Autodesk Inventor part; units mm, degrees
ref_plane "YZ Plane" through (0, 0, 0) normal (1, 0, 0) x (0, 1, 0)
ref_plane "XZ Plane" through (0, 0, 0) normal (0, 1, 0) x (-1, 0, 0)
ref_plane "XY Plane" through (0, 0, 0) normal (0, 0, 1) x (1, 0, 0)
ref_plane "Plano de trabajo1" through (0, 3, 0) normal (0, 1, 0) x (1, 0, 0)
ref_plane "Plano de trabajo2" through (4.2498, 73, -5.25) normal (0, 1, 0) x (1, 0, 0)
sketch "Boceto3" plane through (4.2498, 73, -5.25) normal (0, 1, 0) x (1, 0, 0)
  line L0 (37.7502, 51.75) -> (40.7502, 51.75)
  line L1 (-7.2498, -8.25) -> (40.7502, -8.25)
  line L2 (40.7502, -8.25) -> (40.7502, 51.75)
  line L3 (40.7502, 51.75) -> (-7.2498, 51.75)
  line L4 (-7.2498, 51.75) -> (-7.2498, -8.25)
  circle A0 centre (33.5, 43.5) radius 1.25
  circle A1 centre (33.5, 0) radius 1.25
  circle A2 centre (0, 43.5) radius 1.25
  circle A3 centre (0, 0) radius 1.25
  point P0 (-4.2498, -5.25)
  point P1 (37.7502, -5.25)
  point P2 (37.7502, 48.75)
  dimension "d39" = 2.5
  dimension "d40" = 2.5
  dimension "d41" = 2.5
  dimension "d42" = 2.5
ref_plane "Plano de trabajo3" through (4.2498, 73, -5.25) normal (0, -1, 0) x (1, 0, 0)
sketch "Boceto5" plane through (4.2498, 73, -5.25) normal (0, -1, 0) x (1, 0, 0)
  line L0 (-4.2498, 5.25) -> (-4.2498, -48.75)
  line L1 (-4.2498, 5.25) -> (-4.2498, -48.75)
  line L2 (37.7502, -48.75) -> (37.7502, 5.25)
  line L3 (37.7502, 5.25) -> (37.7502, 8.25)
  line L4 (37.7502, -48.75) -> (37.7502, -51.75)
  line L5 (-4.2498, 5.25) -> (-7.2498, 5.25)
  line L6 (-4.2498, -48.75) -> (-7.2498, -48.75)
  line L7 (37.7502, -48.75) -> (40.7502, -48.75)
  line L8 (37.7502, 5.25) -> (40.7502, 5.25)
  line L9 (40.7502, 5.25) -> (40.7502, -48.75)
  line L10 (40.7502, -51.75) -> (40.7502, 8.25)
  line L11 (-7.2498, -48.75) -> (-7.2498, 5.25)
  line L12 (-7.2498, 8.25) -> (-7.2498, -51.75)
extrude "Extrusión5" add sketch "Boceto5" along normal blind 67.5
extrude "Extrusión6" add sketch "Boceto3" along normal blind 3
sketch "Boceto6" plane through (4.2498, 76, -5.25) normal (0, 1, 0) x (1, 0, 0)
  circle A0 centre (0, 43.5) radius 1.25
  circle A1 centre (0, 43.5) radius 1.25
  circle A2 centre (33.5, 43.5) radius 1.25
  circle A3 centre (33.5, 43.5) radius 1.25
  circle A4 centre (33.5, 0) radius 1.25
  circle A5 centre (33.5, 0) radius 1.25
  circle A6 centre (0, 0) radius 1.25
  point P0 (-4.2498, -5.25)
extrude "Extrusión7" add sketch "Boceto6" against normal blind 3
sketch "Boceto8" plane through (45, 5.5, 0) normal (1, 0, 0) x (0, 0, -1)
  line L0 (0, 0) -> (54, 0)
  line L1 (0, 0) -> (54, 0)
  line L2 (54, 0) -> (54, 1.5)
  line L3 (54, 1.5) -> (0, 1.5)
  line L4 (0, 67.5) -> (0, 0)
  line L5 (0, 0) -> (0, 1.5)
  line L6 (54, 1.5) -> (54, 21.5)
  line L7 (54, 21.5) -> (54, 22.5)
  line L8 (54, 22.5) -> (0, 22.5)
  line L9 (0, 22.5) -> (0, 24)
  line L10 (0, 24) -> (54, 24)
  line L11 (54, 22.5) -> (54, 24)
  line L12 (54, 24) -> (54, 45)
  line L13 (54, 67.5) -> (54, 0)
  line L14 (54, 45) -> (0, 45)
  line L15 (0, 45) -> (0, 46.5)
  line L16 (0, 46.5) -> (54, 46.5)
  line L17 (54, 45) -> (54, 46.5)
  line L18 (54, 67.5) -> (0, 67.5)
  line L19 (54, 46.5) -> (54, 67.5)
  point P0 (0, -5.5)
  dimension "d54" = 1.5
  dimension "d55" = 20
  dimension "d60" = 1
  dimension "d61" = 1.5
  dimension "d62" = 21
  dimension "d63" = 1.5
extrude "Extrusión8" add sketch "Boceto8" against normal blind 47.25 contours L4 L3 L2 L0 | L4 L10 L11 L8 | L4 L16 L13 L14
sketch "Boceto9" plane through (-3, 5.5, 0) normal (0, 0, 1) x (1, 0, 0)
  line L0 (3, 67.5) -> (3, 46.5)
  line L1 (3, 46.5) -> (3, 52.5)
  line L2 (3, 52.5) -> (45, 52.5)
  line L3 (45, 67.5) -> (45, 46.5)
  line L4 (45, 52.5) -> (45, 46.5)
  line L5 (45, 46.5) -> (3, 46.5)
  line L6 (45, 46.5) -> (3, 46.5)
  line L7 (45, 45) -> (45, 24)
  line L8 (3, 24) -> (45, 24)
  line L9 (45, 24) -> (45, 30)
  line L10 (45, 30) -> (3, 30)
  line L11 (3, 30) -> (3, 24)
  line L12 (45, 22.5) -> (45, 1.5)
  line L13 (3, 2) -> (3, 1.5)
  line L14 (45, 1.5) -> (3, 1.5)
  line L15 (3, 1.5) -> (45, 1.5)
  line L16 (45, 1.5) -> (45, 7.5)
  line L17 (45, 22.5) -> (45, 1.5)
  line L18 (45, 7.5) -> (3, 7.5)
  line L19 (45, 7.5) -> (45, 1.5)
  line L20 (3, 1.5) -> (3, 7.5)
  line L21 (3, 22.5) -> (3, 1.5)
  point P0 (3, -5.5)
  point P1 (45, 8)
  point P2 (45, 2)
  dimension "d66" = 6
  dimension "d70" = 6
extrude "Extrusión10" add sketch "Boceto9" along normal blind 1.5
sketch "Boceto11" plane through (-3, 5.5, 0) normal (0, 0, 1) x (1, 0, 0)
  line L0 (48, 0) -> (0, 0)
  line L1 (48, 0) -> (0, 0)
  line L2 (0, 0) -> (0, 67.5)
  line L3 (3, 67.5) -> (3, 52.5)
  line L4 (0, 67.5) -> (3, 67.5)
  line L5 (3, 67.5) -> (3, 46.5)
  line L6 (45, 46.5) -> (3, 46.5)
  line L7 (3, 46.5) -> (45, 46.5)
  line L8 (45, 67.5) -> (45, 52.5)
  line L9 (45, 46.5) -> (45, 67.5)
  line L10 (48, 67.5) -> (45, 67.5)
  line L11 (45, 67.5) -> (48, 67.5)
  line L12 (48, 67.5) -> (48, 0)
  line L13 (3, 7.5) -> (3, 1.5)
  line L14 (3, 22.5) -> (3, 7.5)
  line L15 (3, 7.5) -> (3, 22.5)
  line L16 (3, 22.5) -> (45, 22.5)
  line L17 (45, 22.5) -> (45, 1.5)
  line L18 (45, 22.5) -> (45, 1.5)
  line L19 (45, 1.5) -> (3, 1.5)
  line L20 (3, 1.5) -> (3, 7.5)
  line L21 (45, 24) -> (3, 24)
  line L22 (3, 24) -> (45, 24)
  line L23 (45, 24) -> (45, 45)
  line L24 (3, 45) -> (3, 30)
  line L25 (45, 45) -> (3, 45)
  line L26 (3, 45) -> (3, 24)
  point P0 (3, -5.5)
  dimension "d75" = 21
extrude "Extrusión12" add sketch "Boceto11" along normal blind 1.5
sketch "Boceto12" plane through (-3, 73, 3) normal (0, 0, 1) x (1, 0, 0)
  line L0 (45, 0) -> (48, 0)
  line L1 (0, 3) -> (48, 3)
  line L2 (48, 3) -> (48, 0)
  line L3 (48, 0) -> (0, 0)
  line L4 (0, 0) -> (0, 3)
  point P0 (3, -73)
extrude "Extrusión13" cut sketch "Boceto12" against normal blind 1.5
sketch "Boceto13" plane through (45, 73, -57) normal (0, 0, -1) x (-1, 0, 0)
  line L0 (0, 3) -> (48, 3)
  line L1 (48, 3) -> (48, 0)
  line L2 (48, 0) -> (0, 0)
  line L3 (0, 0) -> (0, 3)
  point P0 (45, -73)
extrude "Extrusión14" cut sketch "Boceto13" against normal blind 3
sketch "Boceto14" plane through (-3, 5.5, 1.5) normal (0, 0, 1) x (1, 0, 0)
  line L0 (48, 70.5) -> (0, 70.5)
  line L1 (0, 0) -> (48, 0)
  line L2 (0, 70.5) -> (48, 70.5)
  line L3 (48, 70.5) -> (48, 0)
  line L4 (48, 0) -> (0, 0)
  line L5 (0, 0) -> (0, 70.5)
  line L6 (3, 45) -> (45, 45)
  line L7 (3, 45) -> (45, 45)
  line L8 (45, 45) -> (45, 30)
  line L9 (45, 30) -> (3, 30)
  line L10 (3, 30) -> (3, 45)
  line L11 (3, 22.5) -> (45, 22.5)
  line L12 (45, 22.5) -> (45, 1.5)
  line L13 (3, 22.5) -> (45, 22.5)
  line L14 (45, 22.5) -> (45, 7.5257)
  line L15 (45, 7.5257) -> (3, 7.5257)
  line L16 (3, 7.5257) -> (3, 22.5)
  line L17 (3, 52.5) -> (3, 67.5)
  line L18 (45, 67.5) -> (45, 46.5)
  line L19 (3, 67.5) -> (45, 67.5)
  line L20 (45, 67.5) -> (45, 52.5)
  line L21 (45, 52.5) -> (3, 52.5)
  line L22 (3, 52.5) -> (3, 67.5)
  point P0 (3, -5.5)
  dimension "d86" = 15
extrude "Extrusión15" add sketch "Boceto14" along normal blind 5.5
sketch "Boceto15" plane through (0, 58, 0) normal (0, 1, 0) x (1, 0, 0)
  line L0 (42, 0) -> (42, -7)
  line L1 (0, -7) -> (0, 0)
  line L2 (0, -7) -> (1.5, -7)
  line L3 (0, -7) -> (0, -5.5)
  line L4 (0, 0) -> (0, -7)
  line L5 (42, -7) -> (42, -6)
  line L6 (42, 0) -> (42, -7)
  line L7 (42, -6) -> (0, -6)
  line L8 (0, -7) -> (0, -6)
  line L9 (0, 0) -> (0, -1)
  line L10 (0, -1) -> (42, -1)
  line L11 (42, 0) -> (42, -1)
  dimension "d89" = 1.5
  dimension "d90" = 1.5
  dimension "d91" = 1
extrude "Extrusión16" cut sketch "Boceto15" against normal blind 41.75
sketch "Boceto16" plane through (0, 28, 1) normal (0, 0, 1) x (1, 0, 0)
  line L0 (42, 0) -> (0, 0)
  line L1 (0, 0) -> (42, 0)
  line L2 (0, 7.5) -> (42, 7.5)
  line L3 (21, 0) -> (18.5, 0)
  line L4 (18.5, 0) -> (18.5, 7.5)
  line L5 (18.5, 7.5) -> (23.5, 7.5)
  line L6 (23.5, 7.5) -> (23.5, 0)
  point P0 (0, -28)
  dimension "d94" = 2.5
  dimension "d95" = 5
extrude "Extrusión17" add sketch "Boceto16" along normal blind 5.75
sketch "Boceto17" plane through (0, 58, 1) normal (0, 0, 1) x (1, 0, 0)
  line L0 (0, 0) -> (42, 0)
  line L1 (21, 0) -> (18.5, 0)
  line L2 (18.5, 0) -> (23.5, 0)
  line L3 (23.5, 0) -> (23.5, -7.5)
  line L4 (42, -28.5) -> (0, -28.5)
  line L5 (23.5, -7.5) -> (18.5, -7.5)
  line L6 (42, -7.5) -> (0, -7.5)
  line L7 (18.5, 0) -> (18.5, -7.5)
  point P0 (0, -58)
  dimension "d98" = 2.5
  dimension "d99" = 5
  dimension "d100" = 7.5
extrude "Extrusión18" add sketch "Boceto17" along normal blind 5.75
sketch "Boceto18" plane through (4.2498, 76, -5.25) normal (0, 1, 0) x (1, 0, 0)
  line L0 (-4.2498, 48.75) -> (-4.2498, -12.25)
  line L1 (-4.2498, -12.25) -> (-4.2498, -11.25)
  line L2 (-4.2498, -11.25) -> (-4.2498, -6.25)
  line L3 (2.5002, -11.25) -> (7.5002, -11.25)
  line L4 (-4.2498, -5.25) -> (-4.2498, 48.75)
  line L5 (7.5002, -11.25) -> (7.5002, -6.25)
  line L6 (2.5002, -11.25) -> (2.5002, -6.25)
  line L7 (2.5002, -6.25) -> (7.5002, -6.25)
  line L8 (23.5002, -6.25) -> (23.5002, -11.25)
  line L9 (33.5002, -6.25) -> (33.5002, -11.25)
  line L10 (23.5002, -6.25) -> (33.5002, -6.25)
  line L11 (23.5002, -11.25) -> (33.5002, -11.25)
  dimension "d103" = 1
  dimension "d104" = 5
extrude "Extrusión19" cut sketch "Boceto18" against normal blind 6
sketch "Boceto19" plane through (4.2498, 76, -5.25) normal (0, 1, 0) x (1, 0, 0)
  line L0 (23.5002, -6.25) -> (33.5002, -6.25)
  line L1 (23.5002, -6.25) -> (22.2502, -6.25)
  line L2 (37.7502, -6.25) -> (19.2502, -6.25)
  line L3 (23.5002, -11.25) -> (22.2502, -11.25)
  line L4 (19.2502, -11.25) -> (37.7502, -11.25)
  line L5 (22.2502, -6.25) -> (22.2502, -11.25)
  line L6 (-4.2498, -6.75) -> (37.7502, -6.75)
  line L7 (33.5002, -6.25) -> (35, -6.25)
  line L8 (35, -11.25) -> (35, -6.25)
  line L9 (23.5002, -11.25) -> (33.5002, -11.25)
  line L10 (35, -11.25) -> (33.5002, -11.25)
  point P0 (-4.2498, -5.25)
  dimension "d115" = 1.25
extrude "Extrusión20" cut sketch "Boceto19" against normal blind 9.5
sketch "Boceto20" plane through (-3, 5.5, 7) normal (0, 0, 1) x (1, 0, 0)
  line L0 (3, 7.5) -> (3, 7.5257)
  line L1 (45, 1.5) -> (3, 1.5)
  line L2 (4.2634, 4.6029) -> (9.2628, 4.6029)
  line L3 (4.2634, 2.9329) -> (9.2628, 2.9329)
  line L4 (4.2634, 3.1329) -> (9.2628, 3.1329)
  line L5 (4.2634, 4.8029) -> (9.2628, 4.8029)
  line L6 (4.2634, 4.8029) -> (4.2634, 6.2729)
  line L7 (4.2634, 6.2729) -> (9.2628, 6.2729)
  line L8 (9.2628, 2.9329) -> (9.2628, 1.4629)
  line L9 (9.2628, 1.4629) -> (4.2634, 1.4629)
  line L10 (4.2634, 1.4629) -> (4.2634, 2.9329)
  line L11 (4.2634, 3.1329) -> (4.2634, 4.6029)
  line L12 (9.2628, 4.8029) -> (9.2628, 6.2729)
  line L13 (9.2628, 4.6029) -> (9.2628, 3.1329)
  point P0 (3, -5.5)
  dimension "d135" = 1.47
extrude "Extrusión21" cut sketch "Boceto20" against normal blind 1
sketch "Boceto21" plane through (-3, 5.5, 7) normal (0, 0, 1) x (1, 0, 0)
  line L0 (4.2634, 6.2729) -> (9.2628, 6.2729)
  line L1 (4.2634, 6.2729) -> (9.2628, 6.2729)
  line L2 (9.2628, 2.9329) -> (9.2628, 1.4629)
  line L3 (9.2628, 6.2729) -> (9.2628, 1.4629)
  line L4 (9.2628, 1.4629) -> (4.2634, 1.4629)
  line L5 (9.2628, 1.4629) -> (4.2634, 1.4629)
  line L6 (4.2634, 4.8029) -> (4.2634, 6.2729)
  line L7 (4.2634, 1.4629) -> (4.2634, 6.2729)
  line L8 (4.2634, 6.2729) -> (4.0634, 6.2729)
  line L9 (4.0634, 6.2729) -> (4.0634, 1.4629)
  line L10 (45, 1.5) -> (3, 1.5)
  line L11 (4.0634, 1.4629) -> (4.2634, 1.4629)
  line L12 (9.2628, 6.2729) -> (9.2628, 4.8029)
  line L13 (9.2628, 6.2729) -> (9.4628, 6.2729)
  line L14 (9.4628, 6.2729) -> (9.4628, 1.4629)
  line L15 (9.4628, 1.4629) -> (9.2628, 1.4629)
  point P0 (3, -5.5)
  dimension "d138" = 0.2
  dimension "d139" = 0.2
extrude "Extrusión22" cut sketch "Boceto21" against normal blind 1 contours L6 L7 L10 L9 L8 | L13 L14 L10 L2 L3 | L7 L11 L9 L10 | L14 L15 L2 L10
sketch "Boceto22" plane through (-3, 5.5, 7) normal (0, 0, 1) x (1, 0, 0)
  line L0 (4.2634, 4.8029) -> (4.2634, 4.6029)
  line L1 (4.2634, 4.7029) -> (4.7634, 4.7029) construction
  line L2 (4.2634, 4.7029) -> (4.2634, 4.9529)
  line L3 (4.2634, 4.7029) -> (4.2634, 4.4529)
  line L4 (4.2634, 4.4529) -> (9.2628, 4.4529)
  line L5 (4.2634, 4.6029) -> (9.2628, 4.6029)
  line L6 (9.2628, 4.4529) -> (9.2628, 4.9529)
  line L7 (9.2628, 4.6029) -> (9.2628, 4.8029)
  line L8 (9.2628, 4.9529) -> (4.2634, 4.9529)
  line L9 (4.2634, 3.1329) -> (4.2634, 2.9329)
  line L10 (4.2634, 3.0329) -> (4.2634, 3.2829)
  line L11 (4.2634, 3.2829) -> (9.2628, 3.2829)
  line L12 (9.2628, 3.2829) -> (9.2628, 2.7829)
  line L13 (9.2628, 2.7829) -> (4.2634, 2.7829)
  line L14 (4.2634, 2.7829) -> (4.2634, 3.0329)
  point P0 (3, -5.5)
  dimension "d148" = 0.5
  dimension "d149" = 0.25
  dimension "d150" = 0.5
extrude "Extrusión23" add sketch "Boceto22" against normal blind 1
properties part number "Relé - columnes tapa"
Work out the finished part from the listing and answer in its coordinate system (mm). A direction names the side the tool comes from. Give positions to 0.01 mm unless a question says otherwise; leave off trailing zeros. Order: outer loops, then holes, each group sorted by start corner. A loop starts at its lowest first (then second) coordinate and runs counter-clockwise, first axis right, second up. Notation, with made-up numbers: (79, 76) -> (124, 76) arc R15 ccw to (124, 81) -> close; hole circle Ø6 at (12.25, -1.75). An arc over 180 degrees is marked (long way). Answer as a JSON object with one key per item and string values. Group by question number.
1. The mould has two halves that part along X. Classify faces 5 (the flat face through (23.5, 32, 3)), 6 (the flat face through (-3, 40, -24)), 7 (the flat face through (15, 33, 7)): released by +X, released by -X, zero draft, split by the parting line, or undercut.
2. Section A-A on x = 20.5 is taken. Count the separate pieces of the cut face and the enclosed holes in it, plus the area to 3 significant figures.
3. Section B-B on y = 62.5 is taken. Determine the outline of the cut face in (x, z), plus the area to 3 significant figures.
4. Section C-C on z = -12 is taken. Determine the outline of the cut face in (x, y), plus the area to 3 significant figures.
5. Flat-ended cylindrical pins translate along their axes: pin 1 Ø6 at (x, y) = (36, 53.5) entering from -Z; pin 2 Ø3 at (x, y) = (14, 16) entering from +Z; pin 3 Ø2 at (x, y) = (12.5, 33.5) entering from -Z. Find the tip coordinate at first contact, or state that the pin passes through.
6. A tool of negligible diameter and unlimited length cuts with its end or side. For faces 1 (the flat face through (21, 33, 0)), 2 (the flat face through (21, 73, -24)), 3 (the flat face through (39.25, 75, 4)), 4 (the flat face through (18.5, 32, 3)), from which of +Z, -Z, +X, -X, +Y, -Y can it reach the whole face along a straight path? Write none if from no direction.
7. Consider line 1 along Y through (x, z) = (20, 0.5); line 2 along Y through (x, z) = (28, -20); line 3 along Z through (x, y) = (3, 53.5). Determine where each line is inside the solid, lowest interval first. Write a range as [from, to].
Result sheet:
{
 "1": {"face 5": "undercut", "face 6": "released by -X", "face 7": "zero draft"},
 "2": {"separate pieces": "4", "enclosed holes": "0", "area": "584 mm^2"},
 "3": {"outline": "(-3, -54) -> (0, -54) -> (0, 7) -> (-3, 7) -> close; (42, -54) -> (45, -54) -> (45, 7) -> (42, 7) -> close", "area": "366 mm^2"},
 "4": {"outline": "(-3, 5.5) -> (45, 5.5) -> (45, 76) -> (-3, 76) -> close; hole (0, 7) -> (42, 7) -> (42, 28) -> (0, 28) -> close; hole (0, 29.5) -> (42, 29.5) -> (42, 50.5) -> (0, 50.5) -> close; hole (0, 52) -> (42, 52) -> (42, 73) -> (0, 73) -> close", "area": "738 mm^2"},
 "5": {"pin 1": "stops at z = -54", "pin 2": "passes through", "pin 3": "stops at z = 0"},
 "6": {"face 1": "-Z", "face 2": "+Z, -Z", "face 3": "+Y", "face 4": "none"},
 "7": {"line 1": "y = [5.5, 13], [28, 35.5], [50.5, 58], [73, 76]", "line 2": "y = [5.5, 7], [28, 29.5], [50.5, 52], [73, 76]", "line 3": "z = [0, 1], [6, 7]"}
}
